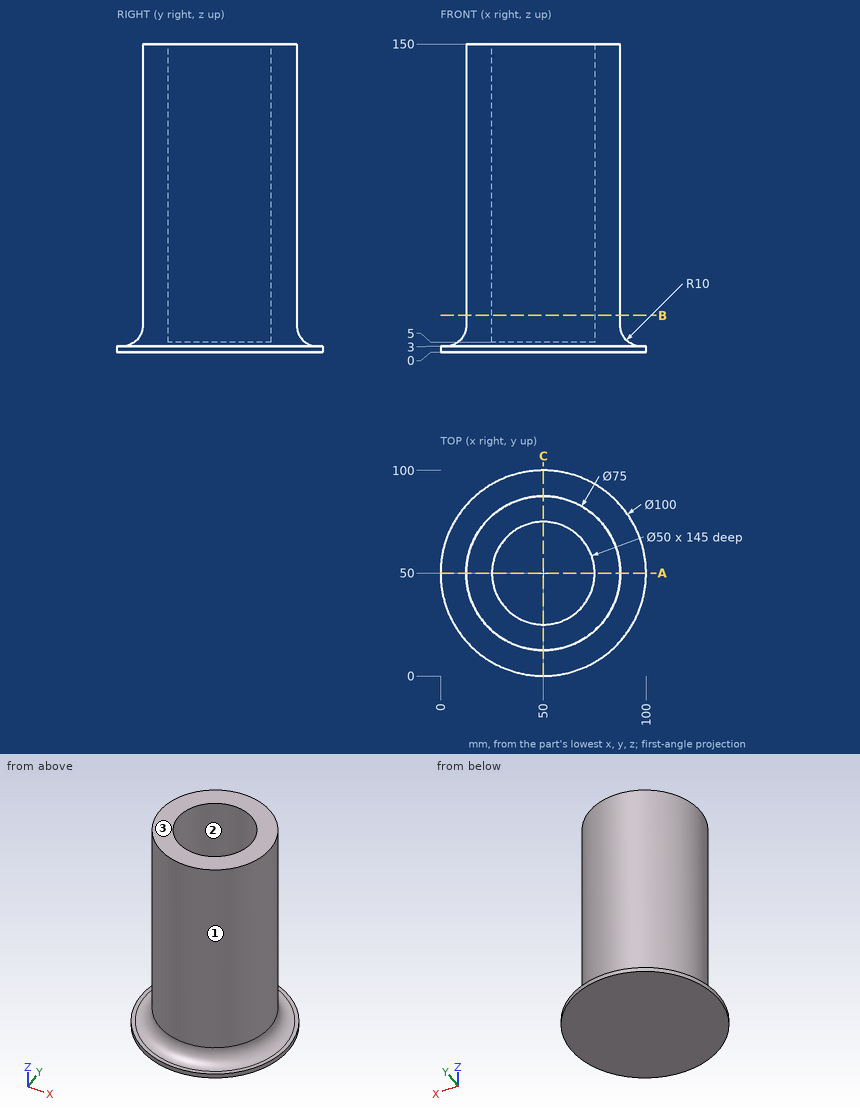
Design review of the part shown in the three views and the two pictorial views. Dimensions are in mm from the part's minimum x, y and z. Round coordinates to 2 decimals unless told otherwise and drop trailing zeros. Loops run counter-clockwise (first coordinate to the right, second up) from the corner with the lowest first, then second, coordinate; pieces in that order, holes last. Notation, with made-up numbers: (-15.75, 58.25) -> (-2.75, 58.25) arc R28 ccw to (-2.75, 96.25) -> close; hole circle Ø2 at (58, 44). An arc over 180 degrees is marked (long way). Answer as a JSON object with one key per item and string values. Group by question number.
1) Mouldability with a two-part tool opening along X and no side actions: class the marked faces 1, 2 and 3 as released by +X, released by -X, zero draft, split by the parting line, or undercut.
2) We need section A-A on y = 50. Write out the cut boundary in (x, z), then the cut area to 3 significant figures.
3) For line 1 (Y direction, x = 50, z = 99.5); line 2 (Z direction, x = 59.5, y = 71); line 3 (Y direction, x = 46, z = 39.5), list the stretches that pass through material, from the lowest coordinate up. Write a range as [from, to].
4) For pin 1 Ø2 at (y, z) = (18.5, 69) entering from +X; pin 2 Ø1 at (x, z) = (58, 97) entering from -Y; pin 3 Ø12 at (x, z) = (62.5, 115.5) entering from +Y; pin 4 Ø8 at (x, y) = (18.5, 76.5) entering from -Z, all flat-tipped, find the tip position at first contact; note any pin that passes through.
5) We need section B-B on z = 18. Write out the cut boundary in (x, y).
Result set:
{
 "1": {"face 1": "split by the parting line", "face 2": "undercut", "face 3": "zero draft"},
 "2": {"outline": "(0, 0) -> (100, 0) -> (100, 3) -> (97.5, 3) arc R10 cw to (87.5, 13) -> (87.5, 150) -> (75, 150) -> (75, 5) -> (25, 5) -> (25, 150) -> (12.5, 150) -> (12.5, 13) arc R10 cw to (2.5, 3) -> (0, 3) -> close", "area": "4,120 mm²"},
 "3": {"line 1": "[12.5, 25], [75, 87.5]", "line 2": "[0, 5]", "line 3": "[12.71, 25.32], [74.68, 87.29]"},
 "4": {"pin 1": "x = 71.82", "pin 2": "y = 13.26", "pin 3": "y = 86.93", "pin 4": "z = 0"},
 "5": {"outline": "circle Ø75 at (50, 50); hole circle Ø50 at (50, 50)"}
}
